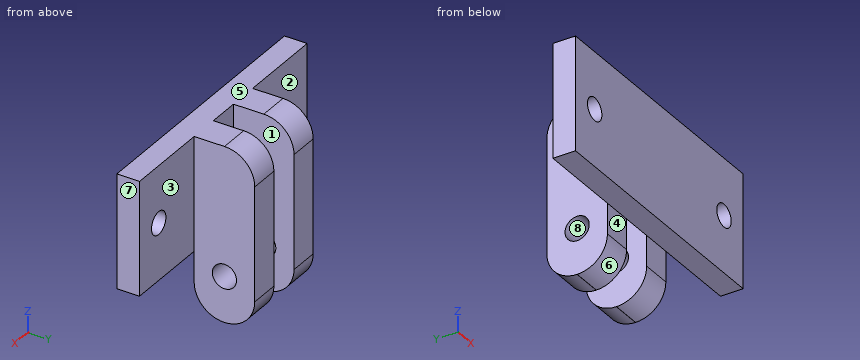
```python
from build123d import *

# Parameters (mm, degrees)
SKETCH1_W           = 35
SKETCH1_H           = 15
BOSS_EXTRUDE1_DEPTH = 3
SKETCH2_W           = 4
SKETCH2_H           = 23
BOSS_EXTRUDE2_DEPTH = 8
SKETCH3_R           = 1.6
CUT_EXTRUDE1_DEPTH  = 8
CUT_EXTRUDE2_START  = -8
SKETCH5_R           = 1.6
CUT_EXTRUDE2_DEPTH  = 8
SKETCH6_R           = 1.5
CUT_EXTRUDE3_DEPTH  = 8


with BuildPart() as part:
    # Sketch1 → Boss-Extrude1 (new body)
    with BuildSketch(Plane(origin=(0, 0, 0), x_dir=(1, 0, 0), z_dir=(0, 1, 0))):
        Rectangle(SKETCH1_W, SKETCH1_H)
    extrude(amount=BOSS_EXTRUDE1_DEPTH)

    # Sketch2 → Boss-Extrude2 (add)
    with BuildSketch(Plane(origin=(0, 3, 0), x_dir=(1, 0, 0), z_dir=(0, 1, 0))):
        with Locations((-4.1, 4)):
            Rectangle(SKETCH2_W, SKETCH2_H)
        with Locations((4.1, 4)):
            Rectangle(SKETCH2_W, SKETCH2_H)
    extrude(amount=BOSS_EXTRUDE2_DEPTH)

    # Sketch3 → Cut-Extrude1 (cut)
    with BuildSketch(Plane.ZY.offset(6.1)):
        with Locations((-9.5, 7)):
            Circle(SKETCH3_R)
        with BuildLine():
            Line((-15.5, 6.99), (-15.5, 3))
            Line((-15.5, 3), (-11.51, 3))
            ThreePointArc((-11.51, 3), (-14.331356057, 4.168643943), (-15.5, 6.99))
        make_face()
        with BuildLine():
            Line((-15.5, 7.01), (-15.5, 11))
            Line((-15.5, 11), (-11.51, 11))
            ThreePointArc((-11.51, 11), (-14.331356057, 9.831356057), (-15.5, 7.01))
        make_face()
        with BuildLine():
            Line((7.5, 11), (7.5, 7.01))
            ThreePointArc((7.5, 7.01), (6.331356057, 9.831356057), (3.51, 11))
            Line((3.51, 11), (7.5, 11))
        make_face()
    extrude(amount=-CUT_EXTRUDE1_DEPTH, mode=Mode.SUBTRACT)

    # Sketch5 → Cut-Extrude2 (cut)
    with BuildSketch(Plane(origin=(6.1, 0, 0), x_dir=(0, 0, -1), z_dir=(1, 0, 0)).offset(CUT_EXTRUDE2_START)):
        with Locations(Location((9.5, 7, 0), (0, 0, 180))):
            Circle(SKETCH5_R)
        with BuildLine():
            Line((11.51, 11), (15.5, 11))
            Line((15.5, 11), (15.5, 7.01))
            ThreePointArc((15.5, 7.01), (14.331356057, 9.831356057), (11.51, 11))
        make_face()
        with BuildLine():
            Line((15.5, 6.99), (15.5, 3))
            Line((15.5, 3), (11.51, 3))
            ThreePointArc((11.51, 3), (14.331356057, 4.168643943), (15.5, 6.99))
        make_face()
        with BuildLine():
            Line((-7.5, 7.01), (-7.5, 11))
            Line((-7.5, 11), (-3.51, 11))
            ThreePointArc((-3.51, 11), (-6.331356057, 9.831356057), (-7.5, 7.01))
        make_face()
    extrude(amount=CUT_EXTRUDE2_DEPTH, mode=Mode.SUBTRACT)

    # Sketch6 → Cut-Extrude3 (cut)
    with BuildSketch(Plane(origin=(0, 3, 0), x_dir=(1, 0, 0), z_dir=(0, 1, 0))):
        with Locations(Location((13.5, 0, 0), (0, 0, 270))):
            Circle(SKETCH6_R)
        with Locations(Location((-13.5, 0, 0), (0, 0, 270))):
            Circle(SKETCH6_R)
    extrude(amount=-CUT_EXTRUDE3_DEPTH, mode=Mode.SUBTRACT)


solid = part.part
```
Geometry check sheet. Reference: the model listing, model coordinates, mm. Face numbers are marked on the shaded views. A direction names the side the tool comes from. Round coordinates to 2 decimals unless told otherwise and drop trailing zeros. Order: outer loops, then holes, each group sorted by start corner. A loop starts at its lowest first (then second) coordinate and runs counter-clockwise, first axis right, second up. Notation, with made-up numbers: (41.25, -3) -> (54.25, -3) arc R34 ccw to (54.25, 30) -> close; hole circle Ø8 at (1, -3.5). An arc over 180 degrees is marked (long way). Return JSON: item names as keys, results as strings. Group by question number.
Q1. Section check A-A, the plane z = 0. Record the boundary of the cut face in (x, y), plus the area to 3 significant figures.
Q2. Material ranges on probe 1 along X at (y, z) = (2, 0); probe 2 along X at (y, z) = (9, -5.75); probe 3 along Z at (x, y) = (3.45, 7), recorded low to high. Write a range as from..to.
Q3. Section check C-C, the plane z = -9.5. Record the boundary of the cut face in (x, y), plus the area to 3 significant figures.
Q4. Release check for a two-part mould opening along Z. For the marked faces 5, 6, 7 and 8 record: released by +Z, released by -Z, zero draft, split by the parting line, or undercut.
Q5. Tool access check on the marked faces 1, 2, 3 and 4. Record the directions out of +Z, -Z, +X, -X, +Y, -Y that give a thin tool (end or side, any length) a straight path to the whole face; none if there is none.
Q6. Section check B-B, the plane x = -13.5. Record the boundary of the cut face in (y, z).
Q7. Gauge pin test, flat ends, axial feed: pin 1 (3 mm diameter, centred on y = 7.5, z = -6.5, fed in from -X); pin 2 (4 mm diameter, centred on x = -3.5, y = 9.5, fed in from +Z); pin 3 (3.5 mm diameter, centred on x = 12.5, z = 1.5, fed in from +Y). Record the tip position at first contact, or that the pin passes through.
Numbers:
{
 "1": {"outline": "(-17.5, 0) -> (-15, 0) -> (-15, 3) -> (-17.5, 3) -> close; (-12, 0) -> (12, 0) -> (12, 3) -> (6.1, 3) -> (6.1, 11) -> (2.1, 11) -> (2.1, 3) -> (-2.1, 3) -> (-2.1, 11) -> (-6.1, 11) -> (-6.1, 3) -> (-12, 3) -> close; (15, 0) -> (17.5, 0) -> (17.5, 3) -> (15, 3) -> close", "area": "151 mm^2"},
 "2": {"probe 1": "-17.5..-15, -12..12, 15..17.5", "probe 2": "-6.1..-2.1, 2.1..6.1", "probe 3": "-15.5..-11.1, -7.9..7.5"},
 "3": {"outline": "(-6.1, 3) -> (-2.1, 3) -> (-2.1, 5.4) -> (-6.1, 5.4) -> close; (-6.1, 8.6) -> (-2.1, 8.6) -> (-2.1, 11) -> (-6.1, 11) -> close; (2.1, 3) -> (6.1, 3) -> (6.1, 5.4) -> (2.1, 5.4) -> close; (2.1, 8.6) -> (6.1, 8.6) -> (6.1, 11) -> (2.1, 11) -> close", "area": "38.4 mm^2"},
 "4": {"face 5": "released by +Z", "face 6": "released by -Z", "face 7": "zero draft", "face 8": "undercut"},
 "5": {"face 1": "+Z, -Z, +Y", "face 2": "+Z, -Z, -X, +Y", "face 3": "+Z, -Z, +X, +Y", "face 4": "-Z, +X, -X, -Y"},
 "6": {"outline": "(0, -7.5) -> (3, -7.5) -> (3, -1.5) -> (0, -1.5) -> close; (0, 1.5) -> (3, 1.5) -> (3, 7.5) -> (0, 7.5) -> close"},
 "7": {"pin 1": "x = -6.1", "pin 2": "z = 7.47", "pin 3": "y = 3"}
}
